Geometry: final body of the model. Coordinates: model frame, mm. Face numbers are marked on the shaded views. A direction names the side the tool comes from. Coordinates: 2 decimals unless noted, no trailing zeros. Loops run counter-clockwise (first coordinate to the right, second up) from the corner with the lowest first, then second, coordinate; pieces in that order, holes last. Notation, with made-up numbers: (-23.5, -12.5) - (-3.5, -12.5) arc R21 ccw to (-3.5, -1.5) - close; hole circle Ø11 at (72.25, -7.75). An arc over 180 degrees is marked (long way). Put each result on its own line as item: value. Start each with the question number.
1) Section D-D on y = -4. Output: boundary loops of the cut face in (x, z) (3 decimals), and give its area (3 significant figures).
2) Material intervals for line 1 along Z through (x, y) = (0, 6.5); line 2 along Y through (x, z) = (-11, 5.5); line 3 along X through (y, z) = (12, -3.25) (3 decimals), sorted ascending. Write a range as from..to.
3) Section A-A on x = -19.05. Output: boundary loops of the cut face in (y, z), and give its area (3 significant figures).
4) Contact query for flat-ended pins moving along their axis: pin 1 Ø1 at (x, z) = (-2.5, 2) entering from +Y; pin 2 Ø3.5 at (x, z) = (-3.5, -0.5) entering from -Y; pin 3 Ø2 at (x, y) = (-42, 16.5) entering from +Z; pin 4 Ø2 at (x, y) = (-18, 2.5) entering from -Z. Output: stop coordinate, or through.
5) Section C-C on x = -9. Output: boundary loops of the cut face in (y, z).
6) Draft query along Z for the marked faces 1, 2 and 3. Return one class per face: +Z half, -Z half, draft (parallel to the pull), parting line (faces both ways), or undercut.
7) Section B-B on y = 17.5. Output: boundary loops of the cut face in (x, z).
8) Reachability of the marked faces 4, 5, 6, 7 and 8 from +Z, -Z, +X, -X, +Y, -Y: full face, straight path, thin tool, end or side. Return the list, or none.
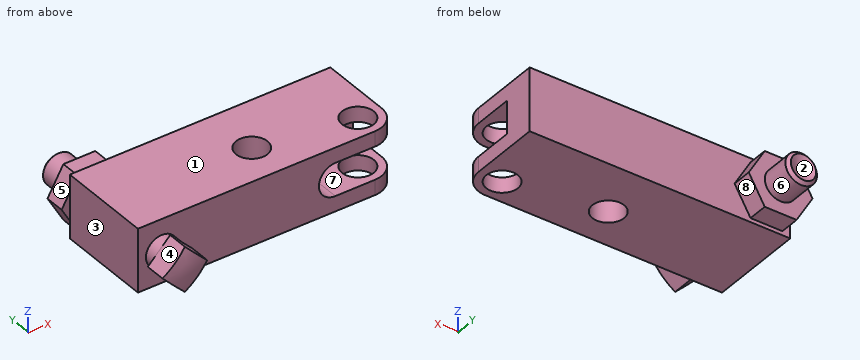
```python
from build123d import *

# Parameters (mm, degrees)
SKETCH11_W         = 52.3748
SKETCH11_H         = 19.05
SKETCH11_R         = 3.1877
SKETCH11_R_2       = 3.18135
EXTRUDE3_DEPTH     = 6.35
CUT_EXTRUDE1_DEPTH = 12.7
FILLET1_R          = 4.7498
EXTRUDE4_DEPTH     = 3.9624
SKETCH15_R         = 10.473643108
CUT_EXTRUDE2_DEPTH = 5.7498


with BuildPart() as part:
    # Sketch11 → Extrude3 (new body, symmetric)
    with BuildSketch(Plane.XY):
        with Locations((-21.4376, 4.7752)):
            Rectangle(SKETCH11_W, SKETCH11_H)
        Circle(SKETCH11_R, mode=Mode.SUBTRACT)
        with Locations((-19.05, 3.175)):
            Circle(SKETCH11_R_2, mode=Mode.SUBTRACT)
    extrude(amount=EXTRUDE3_DEPTH, both=True)

    # Sketch12 → Cut-Extrude1 (cut)
    with BuildSketch(Plane.XZ.offset(4.7498)):
        with BuildLine():
            Line((-7.9502, 3.302), (4.7498, 3.302))
            Line((4.7498, 3.302), (4.7498, -3.302))
            Line((4.7498, -3.302), (-7.9502, -3.302))
            ThreePointArc((-7.9502, -3.302), (-11.2522, 0), (-7.9502, 3.302))
        make_face()
    extrude(amount=-CUT_EXTRUDE1_DEPTH, mode=Mode.SUBTRACT)

    # Fillet1
    fillet1_edges = [part.edges().sort_by_distance(p)[0] for p in [
        (4.7498, -4.7498, -4.826),
        (4.7498, -4.7498, 4.826),
    ]]
    fillet(fillet1_edges, radius=FILLET1_R)

    # Sketch13 → Extrude4 (add)
    with BuildSketch(Plane(origin=(0, 14.3002, 0), x_dir=(1, 0, 0), z_dir=(0, 1, 0))):
        Polygon((-36.441327482, 0), (-39.645563741, 5.5499), (-46.054036259, 5.5499), (-49.258272518, 0), (-46.054036259, -5.5499), (-39.645563741, -5.5499), align=None)
    extrude(amount=EXTRUDE4_DEPTH)

    # Sketch14 → Revolve2 (revolve)
    with BuildSketch(Plane.XY):
        with BuildLine():
            Line((-42.8498, 23.171530316), (-45.3898, 24.638))
            Line((-45.3898, 24.638), (-46.0248, 24.003))
            Line((-46.0248, 24.003), (-46.0248, -7.112))
            Line((-46.0248, -7.112), (-53.323443108, -7.112))
            Line((-53.323443108, -7.112), (-53.323443108, -7.874))
            ThreePointArc((-53.323443108, -7.874), (-48.453364687, -10.831121998), (-42.8498, -11.8618))
            Line((-42.8498, -11.8618), (-42.8498, 23.171530316))
        make_face()
    revolve(axis=Axis((-42.8498, 26.585218564, 0), (0, -1, 0)))

    # Sketch15 → Cut-Extrude2 (cut, through all)
    with BuildSketch(Plane(origin=(0, -7.112, 0), x_dir=(1, 0, 0), z_dir=(0, 1, 0))):
        with Locations((-42.8498, 0)):
            Circle(SKETCH15_R)
        Polygon((-42.8498, 4.490128061), (-47.339928061, 0), (-42.8498, -4.490128061), (-38.359671939, 0), align=None, mode=Mode.SUBTRACT)
    extrude(amount=-CUT_EXTRUDE2_DEPTH, mode=Mode.SUBTRACT)


solid = part.part
```
Answer block:
1. outline: (-47.625, -6.35) - (2.561, -6.35) - (2.561, -3.302) - (-7.95, -3.302) arc R3.302 cw to (-7.95, 3.302) - (2.561, 3.302) - (2.561, 6.35) - (-47.625, 6.35) - close
1. area: 551 mm²
2. line 1: z = -6.35..-3.3, 3.3..6.35
2. line 2: y = -4.75..14.3
2. line 3: x = -47.625..4.75
3. outline: (-4.75, -6.35) - (-0.01, -6.35) - (-0.01, 6.35) - (-4.75, 6.35) - close; (6.36, -6.35) - (14.3, -6.35) - (14.3, 6.35) - (6.36, 6.35) - close
3. area: 161 mm²
4. pin 1: stops at y = 14.3
4. pin 2: stops at y = 7.95
4. pin 3: stops at z = 5.55
4. pin 4: passes through
5. outline: (-4.75, -6.35) - (14.3, -6.35) - (14.3, 6.35) - (-4.75, 6.35) - (-4.75, 3.13) - (7.95, 3.13) - (7.95, -3.13) - (-4.75, -3.13) - close
6. face 1: +Z half
6. face 2: undercut
6. face 3: draft
7. outline: (-49.26, 0) - (-46.05, -5.55) - (-39.65, -5.55) - (-36.44, 0) - (-39.65, 5.55) - (-46.05, 5.55) - close
8. face 4: +Z, -X, -Y
8. face 5: +Z, -X, +Y
8. face 6: +Y
8. face 7: +X, -Y
8. face 8: -Z, +X, +Y
